Check sheet for the modelled part. Datum: model origin and axes. Units: mm. A direction names the side the tool comes from. Give positions to 0.01 mm unless a question says otherwise; leave off trailing zeros. Order: outer loops, then holes, each group sorted by start corner. A loop starts at its lowest first (then second) coordinate and runs counter-clockwise, first axis right, second up.
from build123d import *

# Parameters (mm, degrees)
SKETCH1_R           = 100
SKETCH1_R_2         = 2
SKETCH1_R_3         = 10
BOSS_EXTRUDE1_DEPTH = 5
SKETCH2_R           = 20
SKETCH2_R_2         = 15
BOSS_EXTRUDE2_DEPTH = 6
CUT_EXTRUDE1_REACH  = 143.549
SKETCH3_R           = 1.5


with BuildPart() as part:
    # Sketch1 → Boss-Extrude1 (new body)
    with BuildSketch(Plane.XY):
        Circle(SKETCH1_R)
        with Locations((-32.76709405, -67.463453421)):
            Circle(SKETCH1_R_2, mode=Mode.SUBTRACT)
        with BuildLine():
            ThreePointArc((-18.140194711, -27.362934842), (-31.235810605, -46.349018862), (-47.883759759, -62.311861059))
            ThreePointArc((-47.883759759, -62.311861059), (-54.116540013, -65.899401412), (-61.282970137, -66.499630328))
            ThreePointArc((-61.282970137, -66.499630328), (-76.856869776, -50.591887199), (-87.998157845, -31.318217554))
            ThreePointArc((-87.998157845, -31.318217554), (-89.471065891, -25.164589135), (-88.884816772, -18.864357964))
            ThreePointArc((-88.884816772, -18.864357964), (-85.565152522, -15.829659751), (-81.277194651, -14.472095285))
            ThreePointArc((-81.277194651, -14.472095285), (-62.213907679, -18.258685792), (-42.975567969, -15.495813542))
            ThreePointArc((-42.975567969, -15.495813542), (-33.830845233, -13.716750405), (-24.525208658, -14.159635821))
            ThreePointArc((-24.525208658, -14.159635821), (-17.925326288, -19.113504773), (-18.140194711, -27.362934842))
        make_face(mode=Mode.SUBTRACT)
        with Locations((-74.808611515, -5.354590855)):
            Circle(SKETCH1_R_2, mode=Mode.SUBTRACT)
        with Locations((-18.706228616, -46.368922901)):
            Circle(SKETCH1_R_2, mode=Mode.SUBTRACT)
        with Locations((-14.100447384, -32.034003552)):
            Circle(SKETCH1_R_2, mode=Mode.SUBTRACT)
        with Locations((-49.509779486, -6.98439226)):
            Circle(SKETCH1_R_2, mode=Mode.SUBTRACT)
        with Locations((-34.792484553, -3.805656136)):
            Circle(SKETCH1_R_2, mode=Mode.SUBTRACT)
        with BuildLine():
            ThreePointArc((14.62689934, -29.39133687), (24.521522472, -50.225514922), (30.021774754, -72.62448291))
            ThreePointArc((30.021774754, -72.62448291), (30.012285711, -79.815999122), (26.948884138, -86.322424122))
            ThreePointArc((26.948884138, -86.322424122), (5.385424652, -91.85594528), (-16.876706919, -91.867748957))
            ThreePointArc((-16.876706919, -91.867748957), (-22.942359479, -90.066510532), (-28.105395163, -86.408688317))
            ThreePointArc((-28.105395163, -86.408688317), (-29.073688784, -82.016425638), (-28.105395163, -77.624162959))
            ThreePointArc((-28.105395163, -77.624162959), (-15.294468104, -63.008167415), (-8.068015805, -44.965840374))
            ThreePointArc((-8.068015805, -44.965840374), (-5.036368308, -36.156746606), (0, -28.319271641))
            ThreePointArc((0, -28.319271641), (7.590117545, -25.080540323), (14.62689934, -29.39133687))
        make_face(mode=Mode.SUBTRACT)
        with Locations((42.041517465, -62.108862566)):
            Circle(SKETCH1_R_2, mode=Mode.SUBTRACT)
        with Locations((20.692037169, -28.228347416)):
            Circle(SKETCH1_R_2, mode=Mode.SUBTRACT)
        with Locations((30.80355087, -39.384530641)):
            Circle(SKETCH1_R_2, mode=Mode.SUBTRACT)
        with BuildLine():
            ThreePointArc((32.76709405, -2.028402028), (55.757333077, -3.876496061), (77.905534514, -10.312621851))
            ThreePointArc((77.905534514, -10.312621851), (84.128825724, -13.91659771), (88.231854275, -19.822793794))
            ThreePointArc((88.231854275, -19.822793794), (82.242294427, -41.264058082), (71.121450925, -60.549531403))
            ThreePointArc((71.121450925, -60.549531403), (66.528706412, -64.901921398), (60.779421608, -67.544330353))
            ThreePointArc((60.779421608, -67.544330353), (56.491463738, -66.186765887), (53.171799488, -63.152067674))
            ThreePointArc((53.171799488, -63.152067674), (46.919439575, -44.749481623), (34.907552164, -29.470026832))
            ThreePointArc((34.907552164, -29.470026832), (28.794476925, -22.439996201), (24.525208658, -14.159635821))
            ThreePointArc((24.525208658, -14.159635821), (25.515443833, -5.96703555), (32.76709405, -2.028402028))
        make_face(mode=Mode.SUBTRACT)
        with BuildLine():
            ThreePointArc((-32.76709405, 2.028402028), (-55.757333077, 3.876496061), (-77.905534514, 10.312621851))
            ThreePointArc((-77.905534514, 10.312621851), (-84.128825724, 13.91659771), (-88.231854275, 19.822793794))
            ThreePointArc((-88.231854275, 19.822793794), (-82.242294427, 41.264058082), (-71.121450925, 60.549531403))
            ThreePointArc((-71.121450925, 60.549531403), (-66.528706412, 64.901921398), (-60.779421608, 67.544330353))
            ThreePointArc((-60.779421608, 67.544330353), (-56.491463738, 66.186765887), (-53.171799488, 63.152067674))
            ThreePointArc((-53.171799488, 63.152067674), (-46.919439575, 44.749481623), (-34.907552164, 29.470026832))
            ThreePointArc((-34.907552164, 29.470026832), (-28.794476925, 22.439996201), (-24.525208658, 14.159635821))
            ThreePointArc((-24.525208658, 14.159635821), (-25.515443833, 5.96703555), (-32.76709405, 2.028402028))
        make_face(mode=Mode.SUBTRACT)
        with Locations((-30.80355087, 39.384530641)):
            Circle(SKETCH1_R_2, mode=Mode.SUBTRACT)
        with Locations((-20.692037169, 28.228347416)):
            Circle(SKETCH1_R_2, mode=Mode.SUBTRACT)
        with Locations((-42.041517465, 62.108862566)):
            Circle(SKETCH1_R_2, mode=Mode.SUBTRACT)
        with BuildLine():
            ThreePointArc((-14.62689934, 29.39133687), (-24.521522472, 50.225514922), (-30.021774754, 72.62448291))
            ThreePointArc((-30.021774754, 72.62448291), (-30.012285711, 79.815999122), (-26.948884138, 86.322424122))
            ThreePointArc((-26.948884138, 86.322424122), (-5.385424652, 91.85594528), (16.876706919, 91.867748957))
            ThreePointArc((16.876706919, 91.867748957), (22.942359479, 90.066510532), (28.105395163, 86.408688317))
            ThreePointArc((28.105395163, 86.408688317), (29.073688784, 82.016425638), (28.105395163, 77.624162959))
            ThreePointArc((28.105395163, 77.624162959), (15.294468104, 63.008167415), (8.068015805, 44.965840374))
            ThreePointArc((8.068015805, 44.965840374), (5.036368308, 36.156746606), (0, 28.319271641))
            ThreePointArc((0, 28.319271641), (-7.590117545, 25.080540323), (-14.62689934, 29.39133687))
        make_face(mode=Mode.SUBTRACT)
        with Locations((34.792484553, 3.805656136)):
            Circle(SKETCH1_R_2, mode=Mode.SUBTRACT)
        with Locations((49.509779486, 6.98439226)):
            Circle(SKETCH1_R_2, mode=Mode.SUBTRACT)
        with Locations((14.100447384, 32.034003552)):
            Circle(SKETCH1_R_2, mode=Mode.SUBTRACT)
        with Locations((18.706228616, 46.368922901)):
            Circle(SKETCH1_R_2, mode=Mode.SUBTRACT)
        with Locations((74.808611515, 5.354590855)):
            Circle(SKETCH1_R_2, mode=Mode.SUBTRACT)
        with BuildLine():
            ThreePointArc((18.140194711, 27.362934842), (31.235810605, 46.349018862), (47.883759759, 62.311861059))
            ThreePointArc((47.883759759, 62.311861059), (54.116540013, 65.899401412), (61.282970137, 66.499630328))
            ThreePointArc((61.282970137, 66.499630328), (76.856869776, 50.591887199), (87.998157845, 31.318217554))
            ThreePointArc((87.998157845, 31.318217554), (89.471065891, 25.164589135), (88.884816772, 18.864357964))
            ThreePointArc((88.884816772, 18.864357964), (85.565152522, 15.829659751), (81.277194651, 14.472095285))
            ThreePointArc((81.277194651, 14.472095285), (62.213907679, 18.258685792), (42.975567969, 15.495813542))
            ThreePointArc((42.975567969, 15.495813542), (33.830845233, 13.716750405), (24.525208658, 14.159635821))
            ThreePointArc((24.525208658, 14.159635821), (17.925326288, 19.113504773), (18.140194711, 27.362934842))
        make_face(mode=Mode.SUBTRACT)
        with Locations((32.76709405, 67.463453421)):
            Circle(SKETCH1_R_2, mode=Mode.SUBTRACT)
        Circle(SKETCH1_R_3, mode=Mode.SUBTRACT)
    extrude(amount=BOSS_EXTRUDE1_DEPTH)

    # Sketch2 → Boss-Extrude2 (add)
    with BuildSketch(Plane.XY.offset(5)):
        Circle(SKETCH2_R)
        Circle(SKETCH2_R_2, mode=Mode.SUBTRACT)
    extrude(amount=BOSS_EXTRUDE2_DEPTH)

    # Sketch3 → Cut-Extrude1 (cut, up to next)
    with BuildSketch(Plane.XY.offset(5), mode=Mode.PRIVATE) as cut_extrude1_sk1:
        with Locations((0, 12.5)):
            Circle(SKETCH3_R)
    cut_extrude1_tool1 = extrude(cut_extrude1_sk1.sketch, amount=-CUT_EXTRUDE1_REACH, mode=Mode.PRIVATE) & part.part
    # Sketch3 → Cut-Extrude1 (cut, up to next)
    with BuildSketch(Plane.XY.offset(5), mode=Mode.PRIVATE) as cut_extrude1_sk2:
        with Locations((12.5, 0)):
            Circle(SKETCH3_R)
    cut_extrude1_tool2 = extrude(cut_extrude1_sk2.sketch, amount=-CUT_EXTRUDE1_REACH, mode=Mode.PRIVATE) & part.part
    # Sketch3 → Cut-Extrude1 (cut, up to next)
    with BuildSketch(Plane.XY.offset(5), mode=Mode.PRIVATE) as cut_extrude1_sk3:
        with Locations((0, -12.5)):
            Circle(SKETCH3_R)
    cut_extrude1_tool3 = extrude(cut_extrude1_sk3.sketch, amount=-CUT_EXTRUDE1_REACH, mode=Mode.PRIVATE) & part.part
    # Sketch3 → Cut-Extrude1 (cut, up to next)
    with BuildSketch(Plane.XY.offset(5), mode=Mode.PRIVATE) as cut_extrude1_sk4:
        with Locations((-12.5, 0)):
            Circle(SKETCH3_R)
    cut_extrude1_tool4 = extrude(cut_extrude1_sk4.sketch, amount=-CUT_EXTRUDE1_REACH, mode=Mode.PRIVATE) & part.part
    add(cut_extrude1_tool1.solids().sort_by_distance((0, 12.5, 5))[0], mode=Mode.SUBTRACT)
    add(cut_extrude1_tool2.solids().sort_by_distance((12.5, 0, 5))[0], mode=Mode.SUBTRACT)
    add(cut_extrude1_tool3.solids().sort_by_distance((0, -12.5, 5))[0], mode=Mode.SUBTRACT)
    add(cut_extrude1_tool4.solids().sort_by_distance((-12.5, 0, 5))[0], mode=Mode.SUBTRACT)


solid = part.part
1) Depth check by flat-ended pin: pin 1 Ø2 at (y, z) = (3.5, 6.5) entering from -X; pin 2 Ø3 at (x, y) = (34, -56.5) entering from +Z; pin 3 Ø1.5 at (y, z) = (40, 1.5) entering from +X. Enter the tip coordinate at first touch or a pass-through.
Recorded:
pin 1: stops at x = -19.84
pin 2: stops at z = 5
pin 3: stops at x = 91.98
2) Section check C-C, the plane z = 2.25. State how many separate pieces and enclosed holes the cut face has, then the cut area to 3 significant figures.
Recorded:
separate pieces: 1
enclosed holes: 29
area: 15,400 mm2
3) Section check A-A, the plane x = 66. Record the cut outline in (y, z), then the cut area to 3 significant figures.
Recorded:
outline: (-75.13, 0) - (-65.25, 0) - (-65.25, 5) - (-75.13, 5) - close; (-6.25, 0) - (18.03, 0) - (18.03, 5) - (-6.25, 5) - close; (62.48, 0) - (75.13, 0) - (75.13, 5) - (62.48, 5) - close
area: 234 mm2
4) Set-up check for faces 1 (the face through (-55.44, 3.82, 2.46)), 2 (the face through (3, -10, 5)): record each of +Z, -Z, +X, -X, +Y, -Y from which the full face is reachable in a straight line by a thin tool's end or side.
Recorded:
face 1: +Z, -Z
face 2: +Z
5) Material ranges on L1, parallel to Y at x = 12.5, z = 2.75; L2, parallel to X at y = 35, z = 3.5; L3, parallel to Y at x = -71, z = 3.5, recorded low to high.
Recorded:
L1: y = -99.22 to -90.66, -26.99 to -1.5, 1.5 to 30.83, 33.23 to 57.89, 92.31 to 99.22
L2: x = -93.67 to -84.6, -40.26 to -17.81, 4.45 to 22.73, 86.35 to 93.67
L3: y = -70.42 to -57.54, -17.35 to 7.78, 60.71 to 70.42
6) Draft check along Y on faces 3 (the face through (-15.438, -63.241, 2.465)), 4 (the face through (-24, 1, 5)), 5 (the face through (-56.55, 66.22, 2.46)), 6 (the face through (95.38, 30.04, 2.46)). Enter one of: +Y half, -Y half, draft (parallel to the pull), parting line (faces both ways), or undercut.
Recorded:
face 3: undercut
face 4: draft
face 5: undercut
face 6: parting line
7) Section check B-B, the plane y = 82. Record the cut outline in (x, z).
Recorded:
outline: (-57.24, 0) - (-29.36, 0) - (-29.36, 5) - (-57.24, 5) - close; (29.07, 0) - (57.24, 0) - (57.24, 5) - (29.07, 5) - close
